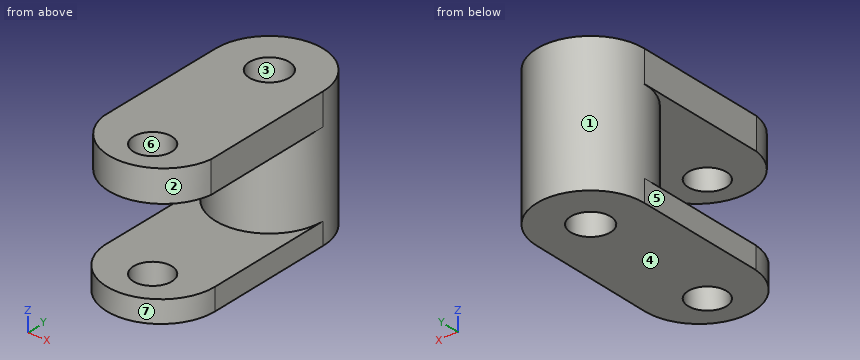
```python
from build123d import *

# Parameters (mm, degrees)
F0_R     = 29.759275958
F1_DEPTH = 76.2
F2_R     = 11.0284850213
F3_DEPTH = 120.142
F5_DEPTH = 12.192
F7_DEPTH = 17.526
F8_R     = 10.6000065129
F9_DEPTH = 148.59


with BuildPart() as f1:
    # F0 (on Top) → F1 (new body)
    with BuildSketch(Plane.XY):
        with Locations((-30.121833086, 0)):
            Circle(F0_R)
    extrude(amount=F1_DEPTH)

    # F2 (on face) → F3 (cut)
    with BuildSketch(Plane.XY.offset(76.2)):
        with Locations((-30.121833086, 0)):
            Circle(F2_R)
    extrude(amount=-F3_DEPTH, mode=Mode.SUBTRACT)

    # F4 (on face) → F5 (join)
    with BuildSketch(Plane(origin=(0, 0, 0), x_dir=(1, 0, 0), z_dir=(0, 0, -1))):
        with BuildLine():
            Line((-59.8811090441, 75.7926106453), (-59.8811090441, 0))
            ThreePointArc((-59.8811090441, 0), (-30.121833086, 29.759275958), (-0.362557128, 0))
            Line((-0.362557128, 0), (0, 73.8646537066))
            ThreePointArc((0, 73.8646537066), (-29.0071131969, 103.8207225337), (-59.8811090441, 75.7926106453))
        make_face()
    extrude(amount=-F5_DEPTH)

    # F6 (on face) → F7 (join)
    with BuildSketch(Plane.XY.offset(76.2)):
        with BuildLine():
            Line((0, -76.4673426747), (-0.362557128, 0))
            ThreePointArc((-0.362557128, 0), (-30.121833086, -29.759275958), (-59.8811090441, 0))
            Line((-59.8811090441, 0), (-59.8811090441, -76.4673426747))
            ThreePointArc((-59.8811090441, -76.4673426747), (-29.940554522, -102.4194670942), (0, -76.4673426747))
        make_face()
    extrude(amount=-F7_DEPTH)

    # F8 (on face) → F9 (cut)
    with BuildSketch(Plane.XY.offset(76.2)):
        with Locations((-27.9265381396, -82.0572450757)):
            Circle(F8_R)
    extrude(amount=-F9_DEPTH, mode=Mode.SUBTRACT)


solid = f1.part
```
Check sheet for the modelled part. Datum: model origin and axes. Units: mm. Face numbers are marked on the shaded views. A direction names the side the tool comes from. Give positions to 0.01 mm unless a question says otherwise; leave off trailing zeros. Order: outer loops, then holes, each group sorted by start corner. A loop starts at its lowest first (then second) coordinate and runs counter-clockwise, first axis right, second up. Notation, with made-up numbers: M -2.5,-4 L 23.5,-4 A26 ccw 23.5,19 Z; hole C 46,-34 d10. An arc over 180 degrees is marked long. Answer in a Markdown table with one row per item. Add a question column.
Q1. Release check for a two-part mould opening along X. For the marked faces 4, 5, 6 and 7 record: released by +X, released by -X, zero draft, split by the parting line, or undercut.
Q2. Gauge pin test, flat ends, axial feed: pin 1 Ø8 at (x, z) = (-23, 18) entering from -Y; pin 2 Ø1.5 at (x, z) = (-45.5, 36) entering from +Y; pin 3 Ø3 at (y, z) = (-90, 13) entering from -X. Record the tip position at first contact, or that the pin passes through.
Q3. Sectioned sample at D-D, the plane y = -59.5. Record the boundary of the cut face in (x, z), and give its area (3 significant figures).
Q4. Sectioned sample at B-B, the plane z = 31. Record the boundary of the cut face in (x, y), and give its area (3 significant figures).
Q5. Sectioned sample at A-A, the plane y = -42. Record the boundary of the cut face in (x, z), and give its area (3 significant figures).
Q6. Thickness scan on L1, parallel to Z at x = -14, y = -71; L2, parallel to Y at x = -27, z = 36; L3, parallel to Y at x = -28.5, z = 50.5. Record the ranges inside material, lowest first.
Q7. Access from +Z, -Z, +X, -X, +Y, -Y to the whole of each face (thin tool, end or side, straight path). Record for the marked faces 1, 2 and 3.
Q8. Sectioned sample at C-C, the plane z = 64. Record the boundary of the cut face in (x, y), and give its area (3 significant figures).
Verdict:
| question | item | result |
|---|---|---|
| 1 | face 4 | zero draft |
| 1 | face 5 | released by -X |
| 1 | face 6 | undercut |
| 1 | face 7 | split by the parting line |
| 2 | pin 1 | y = -29.6 |
| 2 | pin 2 | y = 25.92 |
| 2 | pin 3 | x = -55.99 |
| 3 | outline | M -59.88,0 L -0.07,0 L -0.07,12.19 L -59.88,12.19 Z; M -59.88,58.67 L -0.08,58.67 L -0.08,76.2 L -59.88,76.2 Z |
| 3 | area | 1,780 mm² |
| 4 | outline | C -30.12,0 d59.52; hole C -30.12,0 d22.06 |
| 4 | area | 2,400 mm² |
| 5 | outline | M -59.88,0 L -0.16,0 L -0.16,12.19 L -59.88,12.19 Z; M -59.88,58.67 L -0.16,58.67 L -0.16,76.2 L -59.88,76.2 Z |
| 5 | area | 1,770 mm² |
| 6 | L1 | 0 to 12.19, 58.67 to 76.2 |
| 6 | L2 | -29.6 to -10.58, 10.58 to 29.6 |
| 6 | L3 | -29.72 to -10.91, 10.91 to 29.72 |
| 7 | face 1 | none |
| 7 | face 2 | +Z, -Y |
| 7 | face 3 | +Z, -Z |
| 8 | outline | M -59.88,-76.47 A30.25 ccw 0,-76.47 L -0.36,0 A29.76 ccw -59.88,0 Z; hole C -30.12,0 d22.06; hole C -27.93,-82.06 d21.2 |
| 8 | area | 6,400 mm² |
